Input: part model. Units: mm. Frame: model coordinates. Face numbers are marked on the shaded views. A direction names the side the tool comes from. Round coordinates to 2 decimals unless told otherwise and drop trailing zeros. Order: outer loops, then holes, each group sorted by start corner. A loop starts at its lowest first (then second) coordinate and runs counter-clockwise, first axis right, second up.
Item 1: Reachability of the marked faces 1 and 2 from +Z, -Z, +X, -X, +Y, -Y: full face, straight path, thin tool, end or side. Return the list, or none.
Item 2: Cut plane C-C on y = 39.5. Output: boundary loops of the cut face in (x, z), then the cut area to 4 significant figures.
Item 3: Line query: L1, parallel to X at y = 124.5, z = 18; L2, parallel to Y at x = -71.5, z = 4.5; L3, parallel to X at y = 22.5, z = 14.25. Output: solid intervals per line, ascending.
Item 4: Cut plane A-A on z = 21.75. Give the number of separate pieces and of enclosed holes in the cut face, then the cut area to 3 significant figures.
Item 5: Cut plane B-B on x = -41. Output: boundary loops of the cut face in (y, z), then the cut area to 3 significant figures.
Item 6: Mould query, pull axis Y, two halves, no side actions, for the marked faces 3, 4, 5 and 6. Classes: released by +Y, released by -Y, zero draft, split by the parting line, or undercut.
Item 7: First-contact query: pin 1 (3 mm diameter, centred on x = -167.5, y = 121, fed in from +Z); pin 2 (1.9 mm diameter, centred on x = -75.5, z = 5.5, fed in from -Y); pin 3 (2.5 mm diameter, centred on x = -5, z = 18, fed in from +Y); pin 4 (10.5 mm diameter, centred on x = -37.5, y = 112.5, fed in from +Z). Flat tips, straight axial feed; report the tip coordinate or a pass-through.
Item 8: Cut plane D-D on x = -156.5. Output: boundary loops of the cut face in (y, z), then the cut area to 3 significant figures.
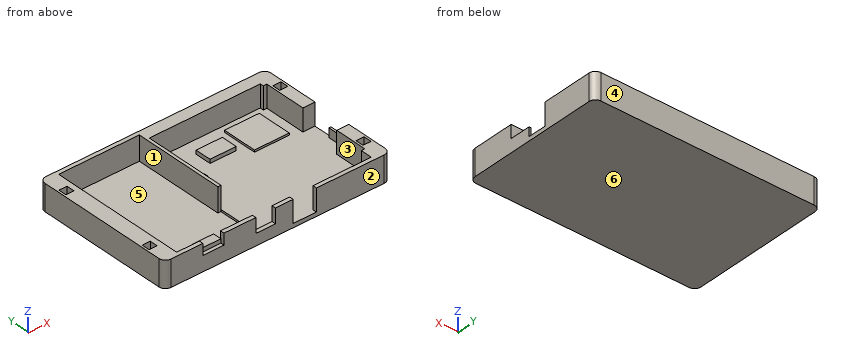
```python
from build123d import *

# Parameters (mm, degrees)
F0_W      = 8
F0_H      = 8
F0_W_2    = 17.6
F0_H_2    = 4
F0_W_3    = 31.5
F0_W_4    = 9.5
F0_H_3    = 37.5
F0_W_5    = 35
F0_H_4    = 34.5
F0_W_6    = 26
F0_H_5    = 15
F0_H_6    = 16
F0_H_7    = 5
F0_W_7    = 12
F0_H_8    = 37
F0_W_8    = 23
F1_DEPTH  = 2
F2_W      = 224
F2_H      = 144
F3_DEPTH  = 24
F4_W      = 21
F4_H      = 4
F5_DEPTH  = 11
F6_W      = 21
F6_H      = 8.5
F7_DEPTH  = 17
F8_R      = 6.35
F9_W      = 34.5
F9_H      = 34.5
F10_DEPTH = 4
F11_W     = 26
F11_H     = 16
F12_DEPTH = 5.8
F14_DEPTH = 4
F15_W     = 19.5
F15_H     = 4
F16_DEPTH = 14.5
F17_W     = 8
F17_H     = 8
F18_DEPTH = 13
F19_W     = 2
F19_H     = 20.5
F20_DEPTH = 13
F21_W     = 2
F21_H     = 18.5
F22_DEPTH = 22
F25_W     = 23
F25_H     = 4
F26_DEPTH = 22
F28_DEPTH = 2


with BuildPart() as f1:
    # F0 (on Top) → F1 (new body)
    with BuildSketch(Plane.XY):
        Polygon((-224, 144), (-224, 0), (-186, 0), (-186, 4), (-208.5, 4), (-208.5, 140), (-128.5, 140), (-128.5, 49.5), (-125.5, 49.5), (-125.5, 87), (-125.5, 132), (-90, 132), (-64, 132), (-15.5, 132), (-15.5, 128.5), (-12, 128.5), (-12, 87), (0, 87), (0, 144), align=None)
        with Locations((-218, 24)):
            Rectangle(F0_W, F0_H, mode=Mode.SUBTRACT)
        with Locations((-218, 120)):
            Rectangle(F0_W, F0_H, mode=Mode.SUBTRACT)
        with Locations((-6, 120)):
            Rectangle(F0_W, F0_H, mode=Mode.SUBTRACT)
        Polygon((-208.5, 4), (-186, 4), (-186, 12), (-165, 12), (-165, 4), (-133.5, 4), (-128.5, 4), (-128.5, 49.5), (-128.5, 140), (-208.5, 140), align=None)
        Polygon((-133.5, 4), (-133.5, 0), (-114, 0), (-114, 4), (-128.5, 4), align=None)
        with Locations((-105.2, 2)):
            Rectangle(F0_W_2, F0_H_2)
        with Locations((-149.25, 2)):
            Rectangle(F0_W_3, F0_H_2)
        Polygon((-186, 4), (-186, 0), (-165, 0), (-165, 4), (-165, 12), (-186, 12), align=None)
        with Locations((-120.75, 68.25)):
            Rectangle(F0_W_4, F0_H_3)
        Polygon((-116, 87), (-12, 87), (-12, 128.5), (-15.5, 128.5), (-15.5, 132), (-64, 132), (-64, 117), (-64, 101), (-64, 96), (-90, 96), (-90, 101), (-90, 117), (-90, 132), (-125.5, 132), (-125.5, 87), align=None)
        with Locations((-39.5, 107.75)):
            Rectangle(F0_W_5, F0_H_4, mode=Mode.SUBTRACT)
        with Locations((-77, 124.5)):
            Rectangle(F0_W_6, F0_H_5)
        with Locations((-77, 109)):
            Rectangle(F0_W_6, F0_H_6)
        with Locations((-77, 98.5)):
            Rectangle(F0_W_6, F0_H_7)
        with Locations((-39.5, 107.75)):
            Rectangle(F0_W_5, F0_H_4)
        with Locations((-6, 120)):
            Rectangle(F0_W, F0_H)
        with Locations((-218, 120)):
            Rectangle(F0_W, F0_H)
        with Locations((-218, 24)):
            Rectangle(F0_W, F0_H)
        with Locations((-6, 68.5)):
            Rectangle(F0_W_7, F0_H_8)
        Polygon((-12, 50), (-12, 87), (-116, 87), (-116, 49.5), (-125.5, 49.5), (-128.5, 49.5), (-128.5, 4), (-114, 4), (-96.4, 4), (-73.4, 4), (-15.5, 4), (-15.5, 15.5), (-12, 15.5), align=None)
        Polygon((0, 0), (0, 50), (-12, 50), (-12, 15.5), (-15.5, 15.5), (-15.5, 4), (-73.4, 4), (-73.4, 0), align=None)
        with Locations((-6, 24)):
            Rectangle(F0_W, F0_H, mode=Mode.SUBTRACT)
        with Locations((-6, 24)):
            Rectangle(F0_W, F0_H)
        with Locations((-84.9, 2)):
            Rectangle(F0_W_8, F0_H_2)
    extrude(amount=F1_DEPTH)

    # F2 (on face) → F3 (join)
    with BuildSketch(Plane.XY.offset(2)):
        with Locations((-112, 72)):
            Rectangle(F2_W, F2_H)
        Polygon((-208.5, 4), (-208.5, 140), (-128.5, 140), (-128.5, 49.5), (-125.5, 49.5), (-125.5, 132), (-15.5, 132), (-15.5, 128.5), (-12, 128.5), (-12, 87), (-2, 87), (-2, 50), (-2, 48), (-12, 48), (-12, 15.5), (-15.5, 15.5), (-15.5, 4), align=None, mode=Mode.SUBTRACT)
    extrude(amount=F3_DEPTH)

    # F4 (on face) → F5 (cut)
    with BuildSketch(Plane.XY.offset(26)):
        with Locations((-175.5, 2)):
            Rectangle(F4_W, F4_H)
    extrude(amount=-F5_DEPTH, mode=Mode.SUBTRACT)

    # F6 (on face) → F7 (join)
    with BuildSketch(Plane.XY.offset(2)):
        with Locations((-175.5, 7.75)):
            Rectangle(F6_W, F6_H)
    extrude(amount=F7_DEPTH)

    # F8
    f8_edges = [f1.edges().sort_by_distance(p)[0] for p in [
        (-224, 0, 13),
        (0, 0, 13),
        (0, 144, 13),
        (-224, 144, 13),
    ]]
    fillet(f8_edges, radius=F8_R)

    # F9 (on face) → F10 (join)
    with BuildSketch(Plane.XY.offset(2)):
        with Locations((-39.75, 107.75)):
            Rectangle(F9_W, F9_H)
    extrude(amount=F10_DEPTH)

    # F11 (on face) → F12 (join)
    with BuildSketch(Plane.XY.offset(2)):
        with Locations((-79, 109)):
            Rectangle(F11_W, F11_H)
    extrude(amount=F12_DEPTH)

    # F13 (on face) → F14 (join)
    with BuildSketch(Plane.XY.offset(2)):
        with BuildLine():
            ThreePointArc((-116, 80.65), (-119.175, 83.825), (-116, 87))
            Line((-116, 87), (-106, 87))
            Line((-106, 87), (-106, 91))
            Line((-106, 91), (-125.5, 91))
            Line((-125.5, 91), (-125.5, 77))
            Line((-125.5, 77), (-116, 77))
            Line((-116, 77), (-116, 80.65))
        make_face()
    extrude(amount=F14_DEPTH)

    # F15 (on face) → F16 (cut)
    with BuildSketch(Plane.XY.offset(26)):
        with Locations((-123.75, 2)):
            Rectangle(F15_W, F15_H)
    extrude(amount=-F16_DEPTH, mode=Mode.SUBTRACT)

    # F17 (on face) → F18 (cut)
    with BuildSketch(Plane.XY.offset(26)):
        with Locations((-218, 120)):
            Rectangle(F17_W, F17_H)
        with Locations((-6, 120)):
            Rectangle(F17_W, F17_H)
        with Locations((-218, 24)):
            Rectangle(F17_W, F17_H)
        with Locations((-6, 24)):
            Rectangle(F17_W, F17_H)
    extrude(amount=-F18_DEPTH, mode=Mode.SUBTRACT)

    # F19 (on face) → F20 (cut)
    with BuildSketch(Plane.XY.offset(26)):
        with Locations((-1, 58.25)):
            Rectangle(F19_W, F19_H)
    extrude(amount=-F20_DEPTH, mode=Mode.SUBTRACT)

    # F21 (on face) → F22 (cut)
    with BuildSketch(Plane.XY.offset(26)):
        with Locations((-1, 77.75)):
            Rectangle(F21_W, F21_H)
    extrude(amount=-F22_DEPTH, mode=Mode.SUBTRACT)

    # F25 (on face) → F26 (cut)
    with BuildSketch(Plane.XY.offset(26)):
        with Locations((-84.9, 2)):
            Rectangle(F25_W, F25_H)
    extrude(amount=-F26_DEPTH, mode=Mode.SUBTRACT)

    # F27 (on face) → F28 (join)
    with BuildSketch(Plane.XY.offset(2)):
        Polygon((-125.5, 132), (-125.5, 4), (-12, 4), (-12, 48), (-2, 48), (-2, 87), (-12, 87), (-12, 132), align=None)
    extrude(amount=F28_DEPTH)


solid = f1.part
```
From the geometry:
1. face 1: +Z
1. face 2: +Z, -Z, +X, -X, -Y
2. outline: (-224, 0) - (0, 0) - (0, 26) - (-12, 26) - (-12, 4) - (-125.5, 4) - (-125.5, 2) - (-208.5, 2) - (-208.5, 26) - (-224, 26) - close
2. area: 1,335 mm2
3. L1: x = -224 to -208.5, -128.5 to -125.5, -12 to 0
3. L2: y = 0 to 4, 101 to 117, 132 to 144
3. L3: x = -224 to -222, -214 to -208.5, -12 to -10, -2 to 0
4. separate pieces: 4
4. enclosed holes: 4
4. area: 5,750 mm2
5. outline: (0, 0) - (144, 0) - (144, 26) - (132, 26) - (132, 4) - (125, 4) - (125, 6) - (90.5, 6) - (90.5, 4) - (4, 4) - (4, 26) - (0, 26) - close
5. area: 997 mm2
6. face 3: undercut
6. face 4: released by +Y
6. face 5: undercut
6. face 6: zero draft
7. pin 1: stops at z = 2
7. pin 2: stops at y = 101
7. pin 3: stops at y = 144
7. pin 4: stops at z = 6
8. outline: (0, 0) - (144, 0) - (144, 26) - (140, 26) - (140, 2) - (4, 2) - (4, 26) - (0, 26) - close
8. area: 480 mm2
